Autodesk Inventor part; units mm, degrees
ref_plane "YZ Plane" through (0, 0, 0) normal (1, 0, 0) x (0, 1, 0)
ref_plane "XZ Plane" through (0, 0, 0) normal (0, 1, 0) x (-1, 0, 0)
ref_plane "XY Plane" through (0, 0, 0) normal (0, 0, 1) x (1, 0, 0)
sketch "Sketch1" plane through (0, 0, 0) normal (0, 0, 1) x (1, 0, 0)
  line L0 (-3.3178, 34.6574) -> (-118.4066, 34.6574)
  line L1 (-118.4066, 34.6574) -> (-118.4066, -30.3526)
  line L2 (-118.4066, -30.3526) -> (-3.3178, -30.3526)
  line L3 (-3.3178, -30.3526) -> (-3.3178, 34.6574)
  line L4 (-118.4066, 17.6954) -> (-127.435, 17.6954)
  line L5 (-127.435, 17.6954) -> (-127.435, 6.6388)
  line L6 (-127.435, 6.6388) -> (-118.4066, 6.6388)
  line L7 (-118.4066, 6.6388) -> (-118.4066, 17.6954)
  line L8 (-118.4066, -17.6281) -> (-127.435, -17.6281)
  line L9 (-127.435, -17.6281) -> (-127.435, -5.7358)
  line L10 (-127.435, -5.7358) -> (-118.4066, -5.7358)
  line L11 (-118.4066, -5.7358) -> (-118.4066, -17.6281)
  line L12 (-3.3178, -17.6281) -> (6.4307, -17.6281)
  line L13 (6.4307, -17.6281) -> (6.4307, -5.7358)
  line L14 (6.4307, -5.7358) -> (-3.3178, -5.7358)
  line L15 (-3.3178, -5.7358) -> (-3.3178, -17.6281)
  line L16 (-3.3178, 17.6954) -> (6.4307, 17.6954)
  line L17 (6.4307, 17.6954) -> (6.4307, 6.1817)
  line L18 (6.4307, 6.1817) -> (-3.3178, 6.1817)
  line L19 (-3.3178, 6.1817) -> (-3.3178, 17.6954)
  point P0 (0, 0)
  point P1 (-3.3178, -5.7358)
  point P2 (-3.3178, 6.1817)
extrude "Extrusion1" add sketch "Sketch1" along normal blind 6
sketch "Sketch2" plane through (0, 0, 6) normal (0, 0, 1) x (1, 0, 0)
  circle A0 centre (-38.1293, 26.639) radius 1.5
  circle A1 centre (-38.1293, -22.361) radius 1.5
  circle A2 centre (-96.1293, -22.361) radius 1.5
  circle A3 centre (-96.1293, 26.639) radius 1.5
  line L0 (6.4307, 17.6954) -> (-3.3178, 17.6954)
  line L1 (-3.3178, 17.6954) -> (-3.3178, 34.6574)
  line L2 (-3.3178, 34.6574) -> (-118.4066, 34.6574)
  line L3 (-118.4066, 34.6574) -> (-118.4066, 17.6954)
  line L4 (-118.4066, 17.6954) -> (-127.435, 17.6954)
  line L5 (-127.435, 17.6954) -> (-127.435, 6.6388)
  line L6 (-127.435, 6.6388) -> (-118.4066, 6.6388)
  line L7 (-118.4066, 6.6388) -> (-118.4066, -5.7358)
  line L8 (-118.4066, -5.7358) -> (-127.435, -5.7358)
  line L9 (-127.435, -5.7358) -> (-127.435, -17.6281)
  line L10 (-127.435, -17.6281) -> (-118.4066, -17.6281)
  line L11 (-118.4066, -17.6281) -> (-118.4066, -30.3526)
  line L12 (-118.4066, -30.3526) -> (-3.3178, -30.3526)
  line L13 (-3.3178, -30.3526) -> (-3.3178, -17.6281)
  line L14 (-3.3178, -17.6281) -> (6.4307, -17.6281)
  line L15 (6.4307, -17.6281) -> (6.4307, -5.7358)
  line L16 (6.4307, -5.7358) -> (-3.3178, -5.7358)
  line L17 (-3.3178, -5.7358) -> (-3.3178, 6.1817)
  line L18 (-3.3178, 6.1817) -> (6.4307, 6.1817)
  line L19 (6.4307, 6.1817) -> (6.4307, 17.6954)
  circle A4 centre (-96.1293, 26.639) radius 2
  circle A5 centre (-96.1293, -22.361) radius 2
  circle A6 centre (-38.1293, -22.361) radius 2
  circle A7 centre (-38.1293, 26.639) radius 2
  point P0 (0, 0)
  dimension "d9" = 4
  dimension "d10" = 4
  dimension "d11" = 4
  dimension "d12" = 4
extrude "Extrusion2" cut sketch "Sketch2" against normal blind 6 contours A0 | A1 | A2 | A3 | A4 | A5 | A6 | A7
sketch "Sketch3" plane through (0, 0, 0) normal (0, 0, -1) x (-1, 0, 0)
  circle A0 centre (-1.5276, 12) radius 1.75
  line L0 (-6.4307, 17.6954) -> (3.3178, 17.6954)
  line L1 (-6.4307, 6.1817) -> (-6.4307, 17.6954)
  line L2 (3.3178, 6.1817) -> (-6.4307, 6.1817)
  line L3 (3.3178, -5.7358) -> (3.3178, 6.1817)
  line L4 (-6.4307, -5.7358) -> (3.3178, -5.7358)
  line L5 (-6.4307, -17.6281) -> (-6.4307, -5.7358)
  line L6 (3.3178, -17.6281) -> (-6.4307, -17.6281)
  line L7 (3.3178, -30.3526) -> (3.3178, -17.6281)
  line L8 (118.4066, -30.3526) -> (3.3178, -30.3526)
  line L9 (118.4066, -17.6281) -> (118.4066, -30.3526)
  line L10 (127.435, -17.6281) -> (118.4066, -17.6281)
  line L11 (127.435, -5.7358) -> (127.435, -17.6281)
  line L12 (118.4066, -5.7358) -> (127.435, -5.7358)
  line L13 (118.4066, 6.6388) -> (118.4066, -5.7358)
  line L14 (127.435, 6.6388) -> (118.4066, 6.6388)
  line L15 (127.435, 17.6954) -> (127.435, 6.6388)
  line L16 (118.4066, 17.6954) -> (127.435, 17.6954)
  line L17 (118.4066, 34.6574) -> (118.4066, 17.6954)
  line L18 (3.3178, 34.6574) -> (118.4066, 34.6574)
  line L19 (3.3178, 17.6954) -> (3.3178, 34.6574)
  circle A1 centre (-1.5276, -12) radius 1.75
  circle A2 centre (122.7276, -12) radius 1.75
  circle A3 centre (122.7276, 12) radius 1.75
  point P0 (0, 0)
extrude "Extrusion3" cut sketch "Sketch3" against normal blind 6 contours A0 | A1 | A2 | A3
sketch "Sketch4" plane through (0, 0, 6) normal (0, 0, 1) x (1, 0, 0)
  circle A0 centre (-38.1293, -22.361) radius 1.5
  circle A1 centre (-96.1293, -22.361) radius 1.5
  circle A2 centre (-38.1293, 26.639) radius 1.5
  circle A3 centre (-96.1293, 26.639) radius 1.5
  arc A4 (-108.1293, -22.361) -> (-100.1293, -30.361) centre (-100.1293, -22.361) ccw
  line L0 (-108.1293, 26.639) -> (-108.1293, -22.361)
  arc A5 (-100.1293, 34.639) -> (-108.1293, 26.639) centre (-100.1293, 26.639) ccw
  line L1 (-21.1293, 34.639) -> (-100.1293, 34.639)
  arc A6 (-13.1293, 26.639) -> (-21.1293, 34.639) centre (-21.1293, 26.639) ccw
  line L2 (-13.1293, -22.361) -> (-13.1293, 26.639)
  arc A7 (-21.1293, -30.361) -> (-13.1293, -22.361) centre (-21.1293, -22.361) ccw
  line L3 (-100.1293, -30.361) -> (-21.1293, -30.361)
  line L4 (-127.435, -17.6281) -> (-118.4066, -17.6281)
  line L5 (-118.4066, -30.3526) -> (-3.3178, -30.3526)
  line L6 (-118.4066, 34.6574) -> (-118.4066, 17.6954)
  line L7 (-118.4066, 17.6954) -> (-104.664, 34.6574)
  line L8 (-3.3178, 34.6574) -> (-118.4066, 34.6574)
  line L9 (-3.3178, 17.6954) -> (-3.3178, 34.6574)
  line L10 (-3.3178, 17.6954) -> (-17.3486, 34.9264)
  line L11 (-3.3178, -17.6281) -> (6.4307, -17.6281)
  line L12 (-109.439, 13.3074) -> (-100.4496, 20.3827)
  line L13 (-100.4496, 20.3827) -> (-26.1151, 20.3827)
  line L14 (-26.1151, 20.3827) -> (-15.4724, 9.6699)
  line L15 (-15.4724, 9.6699) -> (-15.4724, -9.7854)
  line L16 (-15.4724, -9.7854) -> (-22.5627, -16.9004)
  line L17 (-22.5627, -16.9004) -> (-102.211, -16.9004)
  line L18 (-102.211, -16.9004) -> (-109.439, -13.1126)
  line L19 (-109.439, -13.1126) -> (-109.439, 13.3074)
  line L20 (-80.6051, 20.3827) -> (-74.943, 13.3074)
  line L21 (-74.943, 13.3074) -> (-74.943, -8.5904)
  line L22 (-74.943, -8.5904) -> (-80.6051, -16.9004)
  line L23 (-60.8622, 20.3827) -> (-67.4019, 13.1693)
  line L24 (-67.4019, 13.1693) -> (-67.4019, -8.7285)
  line L25 (-67.4019, -8.7285) -> (-60.8622, -16.9004)
  line L26 (-3.3178, -30.3526) -> (-3.3178, -17.6281)
  line L27 (-3.3178, -17.6281) -> (-17.6408, -30.3526)
  line L28 (-118.4066, -30.3526) -> (-3.3178, -30.3526)
  line L29 (-118.4066, -17.6281) -> (-103.6048, -30.3526)
  line L30 (-118.4066, -17.6281) -> (-118.4066, -30.3526)
  line L31 (-118.4066, -17.6281) -> (-118.4066, -30.3526)
  line L32 (-118.4066, -30.3526) -> (-103.6048, -30.3526)
  line L33 (-3.3178, -17.6281) -> (-3.3178, -30.3526)
  line L34 (-17.6408, -30.3526) -> (-3.3178, -30.3526)
  point P0 (0, 0)
  point P1 (-17.1296, 34.6574)
  point P2 (-17.6408, -30.3526)
extrude "Extrusion4" cut sketch "Sketch4" against normal blind 6 contours L27 L26 L5 | L5 L30 L29 | L18 L19 L12 L0 | L0 L12 L13 L20 L21 L22 L17 L18 | L25 L24 L23 L13 L14 L15 L16 L17 | L8 L7 L6 | L8 L9 L10
fillet "Fillet1" radius 5 28 edges at (-127.435, 17.6954, 3) (-127.435, 6.6388, 3) (-127.435, -5.7358, 3) (-127.435, -17.6281, 3) (-104.664, 34.6574, 3) (-17.1296, 34.6574, 3) (6.4307, 17.6954, 3) (6.4307, 6.1817, 3) (6.4307, -5.7358, 3) (6.4307, -17.6281, 3) (-17.6408, -30.3526, 3) (-103.6048, -30.3526, 3) (-80.6051, 20.3827, 3) (-74.943, 13.3074, 3) (-26.1151, 20.3827, 3) (-15.4724, 9.6699, 3) (-15.4724, -9.7854, 3) (-22.5627, -16.9004, 3) (-60.8622, 20.3827, 3) (-67.4019, 13.1693, 3) (-67.4019, -8.7285, 3) (-60.8622, -16.9004, 3) (-109.439, -13.1126, 3) (-102.211, -16.9004, 3) (-100.4496, 20.3827, 3) (-109.439, 13.3074, 3) (-74.943, -8.5904, 3) (-80.6051, -16.9004, 3)
properties part number "Pi_holder"
Here's how the part is built. I have some questions about the finished solid (model axes, mm). A direction names the side the tool comes from. Give positions to 0.01 mm unless a question says otherwise; leave off trailing zeros. Order: outer loops, then holes, each group sorted by start corner. A loop starts at its lowest first (then second) coordinate and runs counter-clockwise, first axis right, second up. Notation, with made-up numbers: (-20, 13) - (25, 13) arc R20 cw to (25, 34) - close; hole circle Ø6 at (13, 17.25). An arc over 180 degrees is marked (long way). Answer as a JSON object with one key per item and string values. Group by question number.
Item 1: If we section it at A-A on x = -86: Please give me the cut outline in (y, z).
Item 2: If we section it at D-D on z = 2.2: Give the number of separate pieces and of enclosed holes in the cut face, and give its area (3 significant figures).
Item 3: If we section it at C-C on x = -64.5: Please give me the cut outline in (y, z).
Item 4: Which directions (+Z, -Z, +X, -X, +Y, -Y) give clear straight access to the entire face, cutting with the end or side of a thin tool? Please do faces 5 (the flat face through (-1, 6.182, 3)), 6 (the flat face through (-105.006, -15.436, 3.042)), 7 (the flat face through (-60, 34.657, 3)).
Item 5: Please list where these lines run through material, in increasing order: probe 1 along Y at (x, z) = (-58.5, 3.2); probe 2 along Y at (x, z) = (-24.5, 1); probe 3 along X at (y, z) = (-21, 3.4).
Item 6: For P1, Ø3, axis at x = -121, z = 2, coming from the +Y side; P2, Ø3, axis at x = -121, z = 3, coming from the -Y side; P3, Ø1, axis at y = -3.5, z = 2, coming from the +X side, each with a flat end and sliding along its axis, tell me the tip position at first contact or that it passes through.
Item 7: If we mould it in two halves opening along X, with no side actions, what happens to faces 1 (the cylindrical face through (4.93, -16.2, 3.04)), 2 (the flat face through (-120, 17.695, 3)), 3 (the flat face through (-118.407, 1, 3)), 4 (the cylindrical face through (-124.397, 12.526, 2.958))? For each: pulls with the +X half, pulls with the -X half, needs draft (parallel to the pull), parting line crosses it, or undercut.
Item 8: If we section it at B-B on y = 2: Please give me the cut outline in (x, z), and give its area (3 significant figures).
Result set:
{
 "1": {"outline": "(-30.35, 0) - (-16.9, 0) - (-16.9, 6) - (-30.35, 6) - close; (20.38, 0) - (34.66, 0) - (34.66, 6) - (20.38, 6) - close"},
 "2": {"separate pieces": "1", "enclosed holes": "10", "area": "4,370 mm²"},
 "3": {"outline": "(-30.35, 0) - (-12.35, 0) - (-12.35, 6) - (-30.35, 6) - close; (16.37, 0) - (34.66, 0) - (34.66, 6) - (16.37, 6) - close"},
 "4": {"face 5": "+Z, -Z, +X", "face 6": "+Z, -Z", "face 7": "+Z, -Z, +X, -X, +Y"},
 "5": {"probe 1": "-30.35 to -16.9, 20.38 to 34.66", "probe 2": "-30.35 to -16.9, 18.76 to 34.66", "probe 3": "-114.48 to -97.59, -94.66 to -39.59, -36.66 to -7.11"},
 "6": {"P1": "y = 17.7", "P2": "y = -17.63", "P3": "x = -3.32"},
 "7": {"face 1": "pulls with the +X half", "face 2": "needs draft", "face 3": "pulls with the -X half", "face 4": "undercut"},
 "8": {"outline": "(-118.41, 0) - (-109.44, 0) - (-109.44, 6) - (-118.41, 6) - close; (-74.94, 0) - (-67.4, 0) - (-67.4, 6) - (-74.94, 6) - close; (-15.47, 0) - (-3.32, 0) - (-3.32, 6) - (-15.47, 6) - close", "area": "172 mm²"}
}
